from build123d import *

# Parameters (mm, degrees)
F1_DEPTH      = 635
F3_DEPTH      = 22
F4_W          = 100
F4_H          = 92
F5_DEPTH      = 10
F6_R          = 11
F7_DEPTH      = 8
F7_DEPTH_BACK = 63.001
F9_DEPTH      = 50.001
F9_DEPTH_BACK = 50.001
F11_DEPTH     = 1
F13_DEPTH     = 1
F14_R         = 10
F15_DEPTH     = 200


with BuildPart() as f1:
    # F0 (on Right) → F1 (new body, symmetric)
    with BuildSketch(Plane.YZ):
        with BuildLine():
            Line((90, 42), (90, 50))
            Line((90, 50), (28, 50))
            ThreePointArc((28, 50), (8.2010101268, 41.7989898732), (0, 22))
            Line((0, 22), (0, -22))
            ThreePointArc((0, -22), (8.2010101268, -41.7989898732), (28, -50))
            Line((28, -50), (90, -50))
            Line((90, -50), (90, -42))
            Line((90, -42), (28, -42))
            ThreePointArc((28, -42), (13.8578643763, -36.1421356237), (8, -22))
            Line((8, -22), (8, 22))
            ThreePointArc((8, 22), (13.8578643763, 36.1421356237), (28, 42))
            Line((28, 42), (90, 42))
        make_face()
    extrude(amount=F1_DEPTH, both=True)

    # F2 (on Top) → F3 (join, symmetric)
    with BuildSketch(Plane.XY):
        Polygon((-80, 0), (-143, 0), (-143, -5), (-85, -5), (-85, -63), (-80, -63), align=None)
        Polygon((80, -63), (85, -63), (85, -5), (143, -5), (143, 0), (80, 0), align=None)
    extrude(amount=F3_DEPTH, both=True)

    # F4 (on face) → F5 (join)
    with BuildSketch(Plane(origin=(0, 90, 0), x_dir=(-1, 0, 0), z_dir=(0, 1, 0))):
        with Locations((-135, 0)):
            Rectangle(F4_W, F4_H)
        with Locations((135, 0)):
            Rectangle(F4_W, F4_H)
    extrude(amount=F5_DEPTH)

    # F6 (on Front) → F7 (cut, two sides)
    with BuildSketch(Plane.XZ) as f7_sk:
        with Locations((-115, 0)):
            Circle(F6_R)
        with Locations((115, 0)):
            Circle(F6_R)
    extrude(amount=-F7_DEPTH, mode=Mode.SUBTRACT)
    extrude(f7_sk.sketch, amount=F7_DEPTH_BACK, mode=Mode.SUBTRACT)

    # F8 (on Top) → F9 (cut, two sides)
    with BuildSketch(Plane.XY) as f9_sk:
        with BuildLine():
            Line((-590, 57.5), (-590, 62.5))
            ThreePointArc((-590, 62.5), (-600, 72.5), (-610, 62.5))
            Line((-610, 62.5), (-610, 57.5))
            ThreePointArc((-610, 57.5), (-600, 47.5), (-590, 57.5))
        make_face()
        with BuildLine():
            ThreePointArc((610, 62.5), (600, 72.5), (590, 62.5))
            Line((590, 62.5), (590, 57.5))
            ThreePointArc((590, 57.5), (600, 47.5), (610, 57.5))
            Line((610, 57.5), (610, 62.5))
        make_face()
    extrude(amount=F9_DEPTH, mode=Mode.SUBTRACT)
    extrude(f9_sk.sketch, amount=-F9_DEPTH_BACK, mode=Mode.SUBTRACT)

    # F10 (on face) → F11 (join)
    with BuildSketch(Plane.XY.offset(50)):
        with BuildLine():
            Line((-582, 57.5), (-582, 62.5))
            ThreePointArc((-582, 62.5), (-600, 80.5), (-618, 62.5))
            Line((-618, 62.5), (-618, 57.5))
            ThreePointArc((-618, 57.5), (-600, 39.5), (-582, 57.5))
        make_face()
        with BuildLine():
            Line((-610, 57.5), (-610, 62.5))
            ThreePointArc((-610, 62.5), (-600, 72.5), (-590, 62.5))
            Line((-590, 62.5), (-590, 57.5))
            ThreePointArc((-590, 57.5), (-600, 47.5), (-610, 57.5))
        make_face(mode=Mode.SUBTRACT)
        with BuildLine():
            Line((618, 57.5), (618, 62.5))
            ThreePointArc((618, 62.5), (600, 80.5), (582, 62.5))
            Line((582, 62.5), (582, 57.5))
            ThreePointArc((582, 57.5), (600, 39.5), (618, 57.5))
        make_face()
        with BuildLine():
            ThreePointArc((610, 57.5), (600, 47.5), (590, 57.5))
            Line((590, 57.5), (590, 62.5))
            ThreePointArc((590, 62.5), (600, 72.5), (610, 62.5))
            Line((610, 62.5), (610, 57.5))
        make_face(mode=Mode.SUBTRACT)
    extrude(amount=F11_DEPTH)

    # F12 (on face) → F13 (join)
    with BuildSketch(Plane.XY.offset(-42)):
        with BuildLine():
            ThreePointArc((-582, 62.5), (-600, 80.5), (-618, 62.5))
            Line((-618, 62.5), (-618, 57.5))
            ThreePointArc((-618, 57.5), (-600, 39.5), (-582, 57.5))
            Line((-582, 57.5), (-582, 62.5))
        make_face()
        with BuildLine():
            Line((-610, 57.5), (-610, 62.5))
            ThreePointArc((-610, 62.5), (-600, 72.5), (-590, 62.5))
            Line((-590, 62.5), (-590, 57.5))
            ThreePointArc((-590, 57.5), (-600, 47.5), (-610, 57.5))
        make_face(mode=Mode.SUBTRACT)
        with BuildLine():
            ThreePointArc((618, 62.5), (600, 80.5), (582, 62.5))
            Line((582, 62.5), (582, 57.5))
            ThreePointArc((582, 57.5), (600, 39.5), (618, 57.5))
            Line((618, 57.5), (618, 62.5))
        make_face()
        with BuildLine():
            ThreePointArc((590, 62.5), (600, 72.5), (610, 62.5))
            Line((610, 62.5), (610, 57.5))
            ThreePointArc((610, 57.5), (600, 47.5), (590, 57.5))
            Line((590, 57.5), (590, 62.5))
        make_face(mode=Mode.SUBTRACT)
    extrude(amount=F13_DEPTH)

    # F14 (on face) → F15 (join)
    with BuildSketch(Plane.XZ.offset(-90)):
        with Locations((-115, 0)):
            Circle(F14_R)
        with Locations((115, 0)):
            Circle(F14_R)
    extrude(amount=F15_DEPTH)


solid = f1.part
Read the model definition and answer for the solid it produces. Units are mm, in the model's axes. A direction names the side the tool comes from. Round coordinates to 2 decimals unless told otherwise and drop trailing zeros. Write each loop counter-clockwise with the first axis right and the second up, starting at its lowest first coordinate (ties: lowest second). Pieces come first, ordered by that corner, then holes. Notation, with made-up numbers: M -13,-9 L 24,-9 A34 cw 24,26 Z; hole C 67.25,49 d5. An arc over 180 degrees is marked long. Use a Markdown table: item, result.
1) Flat-ended cylindrical pins translate along their axes: pin 1 (1 mm diameter, centred on x = -24, z = 8, fed in from -Y); pin 2 (1 mm diameter, centred on y = -74.5, z = -9.5, fed in from -X); pin 3 (8 mm diameter, centred on y = 95, z = 19, fed in from -X). Find the tip coordinate at first contact, or state that the pin passes through.
Answers follow:
| item | result |
|---|---|
| pin 1 | stops at y = 0 |
| pin 2 | stops at x = -119.36 |
| pin 3 | stops at x = -185 |
2) The part is cut by section A-A (y = -19). Write down the section's boundary in (x, z).
Answers follow:
| item | result |
|---|---|
| outline | C -115,0 d20; M -85,-22 L -80,-22 L -80,22 L -85,22 Z; M 80,-22 L 85,-22 L 85,22 L 80,22 Z; C 115,0 d20 |
3) The part is cut by section B-B (x = 47). Write down the section's boundary in (y, z), plus the area to 3 significant figures.
Answers follow:
| item | result |
|---|---|
| outline | M 0,-22 A28 ccw 28,-50 L 90,-50 L 90,-42 L 28,-42 A20 cw 8,-22 L 8,22 A20 cw 28,42 L 90,42 L 90,50 L 28,50 A28 ccw 0,22 Z |
| area | 1,950 mm2 |
4) For a pull along Z with two mould halves and no side action, classify faces 6 (the flat face through (9, 59, -50)), 7 (the cylindrical face through (8.89, 13.703, 35.986)), 8 (the flat face through (-134, 100, 1)) as pulls with the +Z half, pulls with the -Z half, needs draft (parallel to the pull), parting line crosses it, or undercut.
Answers follow:
| item | result |
|---|---|
| face 6 | pulls with the -Z half |
| face 7 | undercut |
| face 8 | needs draft |
5) A tool of negligible diameter and unlimited length cuts with its end or side. For faces 1 (the flat face through (-80, -32, 0)), 2 (the flat face through (-98, -3, 22)), 3 (the cylindrical face through (-126, 1, 0)), 4 (the flat face through (392, 0, 0)), 5 (the cylindrical face through (8.89, 14.014, -36.297)), from which of +Z, -Z, +X, -X, +Y, -Y can it reach the whole face along a straight path? Write none if from no direction.
Answers follow:
| item | result |
|---|---|
| face 1 | +Z, -Z, -Y |
| face 2 | +Z, +X, -X, -Y |
| face 3 | -Y |
| face 4 | +Z, -Z, +X, -Y |
| face 5 | +X, -X |
6) Straight lines are drawn through the part: line 1 along Z through (x, y) = (115, -1); line 2 along Z through (x, y) = (-115, 5); line 3 along Z through (x, y) = (-413.5, 79). For each, find the intervals that lie inside material, in ascending order. Write a range as [from, to].
Answers follow:
| item | result |
|---|---|
| line 1 | z = [-22, -11], [-10, 10], [11, 22] |
| line 2 | z = [-37.97, -11], [-10, 10], [11, 37.97] |
| line 3 | z = [-50, -42], [42, 50] |
